Could you check a few things on this model? Use its own coordinates, in mm. A direction names the side the tool comes from. Coordinates: 2 decimals unless noted, no trailing zeros. Loops run counter-clockwise (first coordinate to the right, second up) from the corner with the lowest first, then second, coordinate; pieces in that order, holes last. Notation, with made-up numbers: (9.25, 61.5) - (18.25, 61.5) arc R35 ccw to (18.25, 100.5) - close; hole circle Ø7 at (-11.75, 52.5). An arc over 180 degrees is marked (long way). Put each result on its own line as item: value. Start each with the question number.
```python
from build123d import *

# Parameters (mm, degrees)
SKETCH1_R           = 7.5
BOSS_EXTRUDE1_DEPTH = 150
SKETCH4_W           = 15
SKETCH4_H           = 30
BOSS_EXTRUDE2_DEPTH = 7.5
SKETCH5_R           = 6
CUT_EXTRUDE2_DEPTH  = 151.934588481


with BuildPart() as part:
    # Sketch1 → Boss-Extrude1 (new body)
    with BuildSketch(Plane.XY):
        Circle(SKETCH1_R)
    extrude(amount=BOSS_EXTRUDE1_DEPTH)

    # Sketch4 → Boss-Extrude2 (add, symmetric)
    with BuildSketch(Plane(origin=(0, 0, 0), x_dir=(1, 0, 0), z_dir=(0, 1, 0))):
        with Locations((0, -15)):
            Rectangle(SKETCH4_W, SKETCH4_H)
    extrude(amount=BOSS_EXTRUDE2_DEPTH, both=True)

    # Sketch5 → Cut-Extrude2 (cut, through all)
    with BuildSketch(Plane(origin=(0, 7.5, 0), x_dir=(1, 0, 0), z_dir=(0, 1, 0))):
        with Locations(Location((0, -15, 0), (0, 0, 270))):
            Circle(SKETCH5_R)
    extrude(amount=-CUT_EXTRUDE2_DEPTH, mode=Mode.SUBTRACT)


solid = part.part
```
(1) For pin 1 Ø1 at (y, z) = (-2.5, 69.5) entering from -X; pin 2 Ø4 at (y, z) = (4.5, 91.5) entering from -X, each with a flat end and sliding along its axis, tell me the tip position at first contact or that it passes through.
(2) I want a section at D-D on z = 119. List the corners of the cut face in (x, y) for me.
(3) I want a section at C-C on y = -3.5. List the corners of the cut face in (x, z) for me, and give its area (3 significant figures).
(4) I want a section at B-B on z = 15. List the corners of the cut face in (x, y) for me.
(5) I need wall thicknesses on L1, parallel to X at y = 2.75, z = 15; L2, parallel to Z at x = 3, y = -2.25; L3, parallel to X at y = -0.25, z = 18.5. Which ranges of each line are inside material? Lowest first, please. Write a range as [from, to].
(6) If we mould it in two halves opening along Z, with no side actions, what happens to faces 1 (the flat face through (0, 0, 0)), 2 (the cylindrical face through (-7.493, 0.33, 89.16)), 3 (the cylindrical face through (-2.3, 0.11, 20.54)), 4 (the flat face through (-6, 6, 30))? For each: pulls with the +Z half, pulls with the -Z half, needs draft (parallel to the pull), parting line crosses it, or undercut.
(7) Which directions (+Z, -Z, +X, -X, +Y, -Y) give clear straight access to the entire face, cutting with the end or side of a thin tool? Please do faces 5 (the flat face through (6, -6, 30)), 6 (the flat face through (0, 0, 150)), 7 (the flat face through (7.5, 0, 15)), 8 (the flat face through (6, 6, 30)), 9 (the flat face through (-6, -6, 30)).
(8) I want a section at A-A on x = 3.5. List the corners of the cut face in (y, z) for me.
Answer sheet:
1. pin 1: stops at x = -7.23
1. pin 2: stops at x = -7.07
2. outline: circle Ø15 at (0, 0)
3. outline: (-7.5, 0) - (7.5, 0) - (7.5, 30) - (6.63, 30) - (6.63, 150) - (-6.63, 150) - (-6.63, 30) - (-7.5, 30) - close; hole circle Ø12 at (0, 15)
3. area: 1,930 mm^2
4. outline: (-7.5, -7.5) - (-6, -7.5) - (-6, 7.5) - (-7.5, 7.5) - close; (6, -7.5) - (7.5, -7.5) - (7.5, 7.5) - (6, 7.5) - close
5. L1: x = [-7.5, -6], [6, 7.5]
5. L2: z = [0, 9.8], [20.2, 150]
5. L3: x = [-7.5, -4.87], [4.87, 7.5]
6. face 1: pulls with the -Z half
6. face 2: needs draft
6. face 3: undercut
6. face 4: pulls with the +Z half
7. face 5: +Z, +X, -Y
7. face 6: +Z, +X, -X, +Y, -Y
7. face 7: +Z, -Z, +X, +Y, -Y
7. face 8: +Z, +X, +Y
7. face 9: +Z, -X, -Y
8. outline: (-7.5, 0) - (7.5, 0) - (7.5, 10.13) - (-7.5, 10.13) - close; (-7.5, 19.87) - (7.5, 19.87) - (7.5, 30) - (6.63, 30) - (6.63, 150) - (-6.63, 150) - (-6.63, 30) - (-7.5, 30) - close
